```python
from build123d import *

# Parameters (mm, degrees)
SKETCH1_W           = 155
SKETCH1_H           = 155
BOSS_EXTRUDE1_DEPTH = 100
SHELL1_T            = -5
SKETCH2_R           = 7.5
CUT_EXTRUDE1_DEPTH  = 5
CUT_EXTRUDE2_REACH  = 202.078
SKETCH5_W           = 145
SKETCH5_H           = 72.5


with BuildPart() as part:
    # Sketch1 → Boss-Extrude1 (new body)
    with BuildSketch(Plane(origin=(0, 0, 0), x_dir=(1, 0, 0), z_dir=(0, 1, 0))):
        Rectangle(SKETCH1_W, SKETCH1_H)
    extrude(amount=BOSS_EXTRUDE1_DEPTH)

    # Shell1
    shell1_openings = [part.faces().sort_by_distance(p)[0] for p in [
        (0, 50, 77.5),
    ]]
    offset(amount=SHELL1_T, openings=shell1_openings, kind=Kind.INTERSECTION)

    # Sketch2 → Cut-Extrude1 (cut)
    with BuildSketch(Plane(origin=(0, 100, 0), x_dir=(1, 0, 0), z_dir=(0, 1, 0))):
        with Locations(Location((0, 0, 0), (0, 0, 270))):
            Circle(SKETCH2_R)
    extrude(amount=-CUT_EXTRUDE1_DEPTH, mode=Mode.SUBTRACT)

    # Cut-Extrude2: up to this face of the body (flat: up to its plane)
    cut_extrude2_end = Plane(part.part.faces().sort_by_distance((77.5, 50, 0))[0])
    # Sketch5 → Cut-Extrude2 (cut, up to the picked face)
    with BuildSketch(Plane.ZY.offset(77.5), mode=Mode.PRIVATE) as cut_extrude2_sk1:
        with Locations((0, 58.75)):
            Rectangle(SKETCH5_W, SKETCH5_H)
    cut_extrude2_tool1 = split(extrude(cut_extrude2_sk1.sketch, amount=-CUT_EXTRUDE2_REACH, mode=Mode.PRIVATE), bisect_by=cut_extrude2_end, keep=Keep.BOTH, mode=Mode.PRIVATE)
    add(cut_extrude2_tool1.solids().sort_by(Axis((-77.5, 58.75, 0), (1, 0, 0)))[0], mode=Mode.SUBTRACT)


solid = part.part
```
Build history of the part. All positions in model axes, mm. A direction names the side the tool comes from. Round coordinates to 2 decimals unless told otherwise and drop trailing zeros. Loops run counter-clockwise (first coordinate to the right, second up) from the corner with the lowest first, then second, coordinate; pieces in that order, holes last.
Item 1: Saw through at D-D (z = 44). List the corners of the cut face in (x, y), then the cut area to 4 significant figures.
Item 2: Saw through at A-A (z = 0). List the corners of the cut face in (x, y).
Item 3: Pin check, flat tip, straight feed: P1, Ø3, axis at x = 23, y = 63.5, coming from the +Z side. Stop position of the tip, or through.
Item 4: Saw through at B-B (x = 0). List the corners of the cut face in (y, z), then the cut area to 4 significant figures.
Item 5: Saw through at C-C (y = 63.5). List the corners of the cut face in (x, z), then the cut area to 3 significant figures.
Item 6: Two-plate mould, pull along X, no slides. Class faces 4 (the face through (-77.5, 20, 0)), 5 (the face through (77.5, 20, 0)), 6 (the face through (0.33, 97.535, -7.493)), 7 (the face through (75, 58, 72.5)): released by +X, released by -X, zero draft, split by the parting line, or undercut.
Item 7: Which spindle directions (+Z, -Z, +X, -X, +Y, -Y) get a long thin tool onto all of the face, cutting with end or side? Do faces 1 (the face through (72.5, 20, 14)), 2 (the face through (-75, 22.5, -1)), 3 (the face through (-1, 49, -77.5)). Say none if no direction does.
Item 8: Drill centre lines: line 1 along Y through (x, z) = (-6.5, -37.5); line 2 along X through (y, z) = (15, 12); line 3 along X through (y, z) = (96, 0). Where is each one in solid material? Low to high.
Worked answers:
1. outline: (-77.5, 0) - (77.5, 0) - (77.5, 22.5) - (72.5, 22.5) - (72.5, 5) - (-72.5, 5) - (-72.5, 22.5) - (-77.5, 22.5) - close; (-77.5, 95) - (77.5, 95) - (77.5, 100) - (-77.5, 100) - close
1. area: 1,725 mm2
2. outline: (-77.5, 0) - (77.5, 0) - (77.5, 22.5) - (72.5, 22.5) - (72.5, 5) - (-72.5, 5) - (-72.5, 22.5) - (-77.5, 22.5) - close; (-77.5, 95) - (-7.5, 95) - (-7.5, 100) - (-77.5, 100) - close; (7.5, 95) - (77.5, 95) - (77.5, 100) - (7.5, 100) - close
3. P1: stops at z = -72.5
4. outline: (0, -77.5) - (100, -77.5) - (100, -7.5) - (95, -7.5) - (95, -72.5) - (5, -72.5) - (5, 77.5) - (0, 77.5) - close; (95, 7.5) - (100, 7.5) - (100, 77.5) - (95, 77.5) - close
4. area: 1,925 mm2
5. outline: (-77.5, -77.5) - (77.5, -77.5) - (77.5, -72.5) - (-77.5, -72.5) - close; (-77.5, 72.5) - (-72.5, 72.5) - (-72.5, 77.5) - (-77.5, 77.5) - close; (72.5, 72.5) - (77.5, 72.5) - (77.5, 77.5) - (72.5, 77.5) - close
5. area: 825 mm2
6. face 4: released by -X
6. face 5: released by +X
6. face 6: undercut
6. face 7: zero draft
7. face 1: +Z
7. face 2: +X, -X
7. face 3: -Z, +X, -X, +Y, -Y
8. line 1: y = 0 to 5, 95 to 100
8. line 2: x = -77.5 to -72.5, 72.5 to 77.5
8. line 3: x = -77.5 to -7.5, 7.5 to 77.5
